from build123d import *

# Parameters (mm, degrees)
F0_W     = 88.9
F0_H     = 44.45
F1_DEPTH = 3.175
F2_R     = 38.608
F2_R_2   = 36.322
F3_DEPTH = 1.524
F5_DEPTH = 3.176


with BuildPart() as f1:
    # F0 (on Top) → F1 (new body)
    with BuildSketch(Plane.XY):
        with Locations((0, -22.225)):
            Rectangle(F0_W, F0_H)
    extrude(amount=F1_DEPTH)

    # F2 (on face) → F3 (cut)
    with BuildSketch(Plane.XY.offset(3.175)):
        Circle(F2_R)
        Circle(F2_R_2, mode=Mode.SUBTRACT)
        with BuildLine():
            Line((-13.208, 0), (13.208, 0))
            ThreePointArc((13.208, 0), (0, 13.208), (-13.208, 0))
        make_face()
        with BuildLine():
            ThreePointArc((-13.208, 0), (0, -13.208), (13.208, 0))
            Line((13.208, 0), (-13.208, 0))
        make_face()
    extrude(amount=-F3_DEPTH, mode=Mode.SUBTRACT)

    # F4 (on Top) → F5 (cut, through all)
    with BuildSketch(Plane.XY):
        with BuildLine():
            ThreePointArc((25.4, 0), (0, 25.4), (-25.4, 0))
            Line((-25.4, 0), (25.4, 0))
        make_face()
        with BuildLine():
            Line((25.4, 0), (-25.4, 0))
            ThreePointArc((-25.4, 0), (0, -25.4), (25.4, 0))
        make_face()
    extrude(amount=F5_DEPTH, mode=Mode.SUBTRACT)


solid = f1.part
Here's how the part is built. I have some questions about the finished solid (model axes, mm). A direction names the side the tool comes from. Coordinates: 2 decimals unless noted, no trailing zeros. Loops run counter-clockwise (first coordinate to the right, second up) from the corner with the lowest first, then second, coordinate; pieces in that order, holes last.
1. Imagine slicing it at B-B, the plane x = 0. Please give me the cut outline in (y, z) (3 decimals).
2. If we mould it in two halves opening along Y, with no side actions, what happens to faces 1 (the flat face through (-1, -44.45, 2)), 2 (the flat face through (-1, -27, 0)), 3 (the cylindrical face through (-0.8, -38.6, 2.4))? For each: pulls with the +Y half, pulls with the -Y half, needs draft (parallel to the pull), parting line crosses it, or undercut.
3. Imagine slicing it at A-A, the plane z = 2.65. Please give me the cut outline in (x, y), and give its area (3 significant figures).
4. I need wall thicknesses on L1, parallel to X at y = -15.5, z = 2.55; L2, parallel to X at y = -10, z = 2.35; L3, parallel to Y at x = -0.5, z = 2.8. Which ranges of each line are inside material? Lowest first, please.
5. Imagine slicing it at D-D, the plane y = -31.5. Please give me the cut outline in (x, z) (3 decimals).
6. For faces 4 (the flat face through (-1, -26, 3.175)), 5 (the cylindrical face through (-0.799, -36.313, 2.424)), which set-ups out of +Z, -Z, +X, -X, +Y, -Y let a thin tool reach every point of the face, with its end or its side?
7. For P1, Ø12, axis at x = -20.5, y = -14.5, coming from the +Z side (3 decimals), with a flat end and sliding along its axis, tell me the tip position at first contact or that it passes through.
8. Imagine slicing it at C-C, the plane y = -11. Please give me the cut outline in (x, z) (3 decimals), and give its area (3 significant figures).
Taken from the geometry:
1. outline: (-44.45, 0) - (-25.4, 0) - (-25.4, 3.175) - (-36.322, 3.175) - (-36.322, 1.651) - (-38.608, 1.651) - (-38.608, 3.175) - (-44.45, 3.175) - close
2. face 1: pulls with the -Y half
2. face 2: needs draft
2. face 3: undercut
3. outline: (-44.45, -44.45) - (44.45, -44.45) - (44.45, 0) - (38.61, 0) arc R38.61 cw to (-38.61, 0) - (-44.45, 0) - close; (-36.32, 0) arc R36.32 ccw to (36.32, 0) - (25.4, 0) arc R25.4 cw to (-25.4, 0) - close
3. area: 2,670 mm2
4. L1: x = -44.45 to -35.36, -32.85 to -20.12, 20.12 to 32.85, 35.36 to 44.45
4. L2: x = -44.45 to -37.29, -34.92 to -23.35, 23.35 to 34.92, 37.29 to 44.45
4. L3: y = -44.45 to -38.6, -36.32 to -25.4
5. outline: (-44.45, 0) - (44.45, 0) - (44.45, 3.175) - (22.323, 3.175) - (22.323, 1.651) - (18.084, 1.651) - (18.084, 3.175) - (-18.084, 3.175) - (-18.084, 1.651) - (-22.323, 1.651) - (-22.323, 3.175) - (-44.45, 3.175) - close
6. face 4: +Z, +X, -X, +Y, -Y
6. face 5: +Z
7. P1: stops at z = 3.175
8. outline: (-44.45, 0) - (-22.895, 0) - (-22.895, 3.175) - (-34.616, 3.175) - (-34.616, 1.651) - (-37.008, 1.651) - (-37.008, 3.175) - (-44.45, 3.175) - close; (22.895, 0) - (44.45, 0) - (44.45, 3.175) - (37.008, 3.175) - (37.008, 1.651) - (34.616, 1.651) - (34.616, 3.175) - (22.895, 3.175) - close
8. area: 130 mm2
